Read the model definition and answer for the solid it produces. Units are mm, in the model's axes. A direction names the side the tool comes from. Coordinates: 2 decimals unless noted, no trailing zeros. Write each loop counter-clockwise with the first axis right and the second up, starting at its lowest first coordinate (ties: lowest second). Pieces come first, ordered by that corner, then holes. Notation, with made-up numbers: M 24,-32 L 71,-32 A20 cw 71,-8 Z; hole C -19.5,88.25 d9. An arc over 180 degrees is marked long. Write item = value, one per line.
from build123d import *

# Parameters (mm, degrees)
SKETCH2_W           = 30
SKETCH2_H           = 120
BOSS_EXTRUDE1_DEPTH = 10
SKETCH3_R           = 1.7
SKETCH3_W           = 20.5
SKETCH3_H           = 40.8
CUT_EXTRUDE3_DEPTH  = 76.224148804


with BuildPart() as part:
    # Sketch2 → Boss-Extrude1 (new body)
    with BuildSketch(Plane.XY):
        with Locations((-15.991735537, -7.809917355)):
            Rectangle(SKETCH2_W, SKETCH2_H)
    extrude(amount=BOSS_EXTRUDE1_DEPTH)

    # Sketch3 → Cut-Extrude3 (cut, through all)
    with BuildSketch(Plane.XY):
        with Locations((-18.291735537, -62.986209282)):
            Circle(SKETCH3_R)
        with Locations((-4.191735537, -62.986209282)):
            Circle(SKETCH3_R)
        with Locations(Location((-4.191735537, -15.786209282, 0), (0, 0, 180))):
            Circle(SKETCH3_R)
        with Locations(Location((-18.291735537, -15.786209282, 0), (0, 0, 180))):
            Circle(SKETCH3_R)
        with Locations((-11.241735537, -39.386209282)):
            Rectangle(SKETCH3_W, SKETCH3_H)
    extrude(amount=CUT_EXTRUDE3_DEPTH, mode=Mode.SUBTRACT)


solid = part.part
Item 1: Find section A-A (x = -11.75). Determine the outline of the cut face in (y, z), and give its area (3 significant figures).
Worked answers:
outline = M -67.81,0 L -59.79,0 L -59.79,10 L -67.81,10 Z; M -18.99,0 L 52.19,0 L 52.19,10 L -18.99,10 Z
area = 792 mm²
Item 2: Consider line 1 along Y through (x, z) = (-3.25, 7); line 2 along Y through (x, z) = (-11, 9.75); line 3 along Y through (x, z) = (-4.75, 1.5). Determine where each line is inside the solid, lowest interval first. Write a range as from..to.
Worked answers:
line_1 = -67.81..-64.4, -61.57..-59.79, -18.99..-17.2, -14.37..52.19
line_2 = -67.81..-59.79, -18.99..52.19
line_3 = -67.81..-64.59, -61.38..-59.79, -18.99..-17.39, -14.18..52.19
Item 3: Find section C-C (y = -22.5). Determine the outline of the cut face in (x, z), and give its area (3 significant figures).
Worked answers:
outline = M -30.99,0 L -21.49,0 L -21.49,10 L -30.99,10 Z
area = 95.0 mm²
Item 4: Find section B-B (z = 2). Determine the outline of the cut face in (x, y), and give its area (3 significant figures).
Worked answers:
outline = M -30.99,-67.81 L -0.99,-67.81 L -0.99,-59.79 L -21.49,-59.79 L -21.49,-18.99 L -0.99,-18.99 L -0.99,52.19 L -30.99,52.19 Z; hole C -18.29,-62.99 d3.4; hole C -18.29,-15.79 d3.4; hole C -4.19,-62.99 d3.4; hole C -4.19,-15.79 d3.4
area = 2,730 mm²
Item 5: For a pull along Y with two mould halves and no side action, classify faces 3 (the face through (-16, -67.81, 5)), 4 (the face through (-11, -59.786, 5)), 5 (the face through (-16, 6, 0)), 6 (the face through (-4.4, -61.3, 4.9)) as released by +Y, released by -Y, zero draft, split by the parting line, or undercut.
Worked answers:
face_3 = released by -Y
face_4 = undercut
face_5 = zero draft
face_6 = undercut
Item 6: Which of the six approach directions +Z, -Z, +X, -X, +Y, -Y give full straight-line access (tool end or side, diameter ignored) to faces 1 (the face through (-21.492, -40, 5)), 2 (the face through (-0.992, -64, 5))?
Worked answers:
face_1 = +Z, -Z, +X
face_2 = +Z, -Z, +X, +Y, -Y
Item 7: Flat-ended cylindrical pins translate along their axes: pin 1 (1 mm diameter, centred on y = -22, z = 6.5, fed in from +X); pin 2 (2.5 mm diameter, centred on x = -4.19, y = -62.99, fed in from -Z); pin 3 (5.5 mm diameter, centred on x = -18.29, y = -62.99, fed in from +Z). Find the tip coordinate at first contact, or state that the pin passes through.
Worked answers:
pin_1 = -21.49
pin_2 = through
pin_3 = 10
